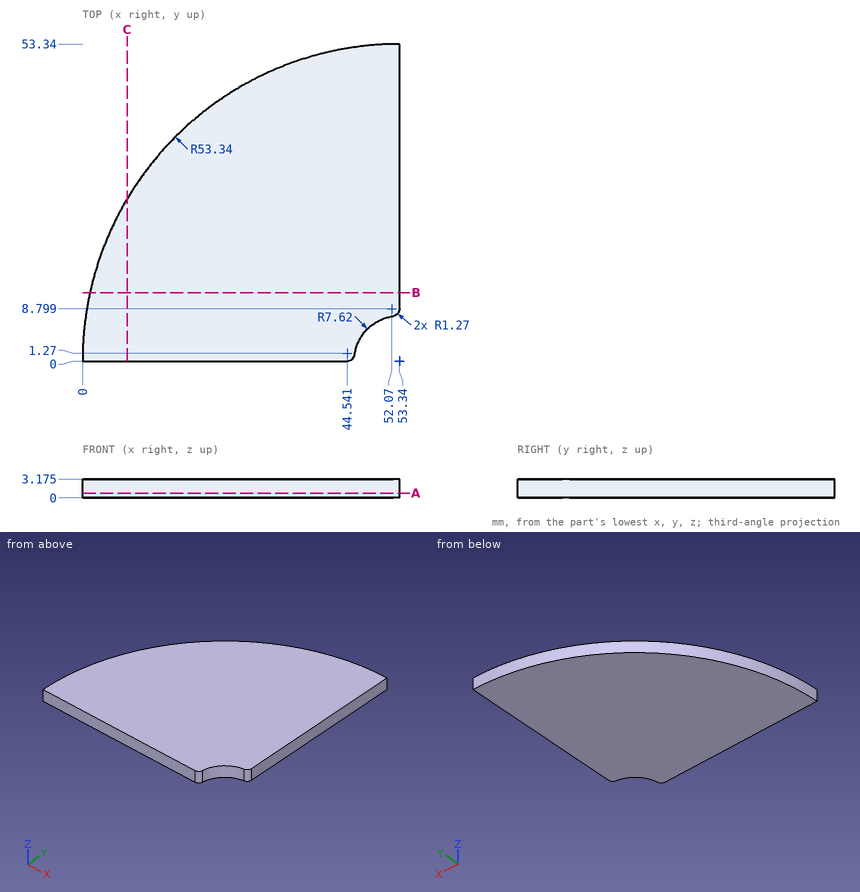
Source: three-view drawing plus pictorial views. Frame: mm from the lowest corner of the part. Give positions to 0.01 mm unless a question says otherwise; leave off trailing zeros. Order: outer loops, then holes, each group sorted by start corner. A loop starts at its lowest first (then second) coordinate and runs counter-clockwise, first axis right, second up. Notation, with made-up numbers: M 19,41.5 L 33,41.5 A23 cw 33,75.5 Z; hole C 56,49 d8. An arc over 180 degrees is marked long. One line per question, with ' | ' between items. Start each with the question number.
1. Section query C-C (x = 7.5). Return the cut outline in (y, z) (1 decimal).
2. Material intervals for probe 1 along Y at (x, z) = (39, 1.7); probe 2 along Y at (x, z) = (5.5, 1.55); probe 3 along X at (y, z) = (14, 2.7), sorted ascending. Write a range as [from, to].
3. Section query A-A (z = 0.8). Return the cut outline in (x, y), and give its area (3 significant figures).
4. Section query B-B (y = 11.5). Return the cut outline in (x, z) (1 decimal).
Here are the results:
1) outline: M 0,0 L 27.3,0 L 27.3,3.2 L 0,3.2 Z
2) probe 1: [0, 51.38] | probe 2: [0, 23.59] | probe 3: [1.87, 53.34]
3) outline: M 0,0 L 44.54,0 A1.27 ccw 45.8,1.09 A7.62 cw 52.25,7.54 A1.27 ccw 53.34,8.8 L 53.34,53.34 A53.34 ccw Z | area: 2,190 mm²
4) outline: M 1.3,0 L 53.3,0 L 53.3,3.2 L 1.3,3.2 Z
